For this review, use the dimensioned drawing (mm, ordinates from the lowest corner) and the shaded views. A direction names the side the tool comes from. Give positions to 0.01 mm unless a question says otherwise; leave off trailing zeros. Loops run counter-clockwise (first coordinate to the right, second up) from the corner with the lowest first, then second, coordinate; pieces in that order, holes last. Notation, with made-up numbers: M 64.25,-14.5 L 112.25,-14.5 A19 ccw 112.25,15.5 Z; hole C 39.25,-30.75 d1. An arc over 180 degrees is marked long. Return JSON: item names as keys, results as strings.
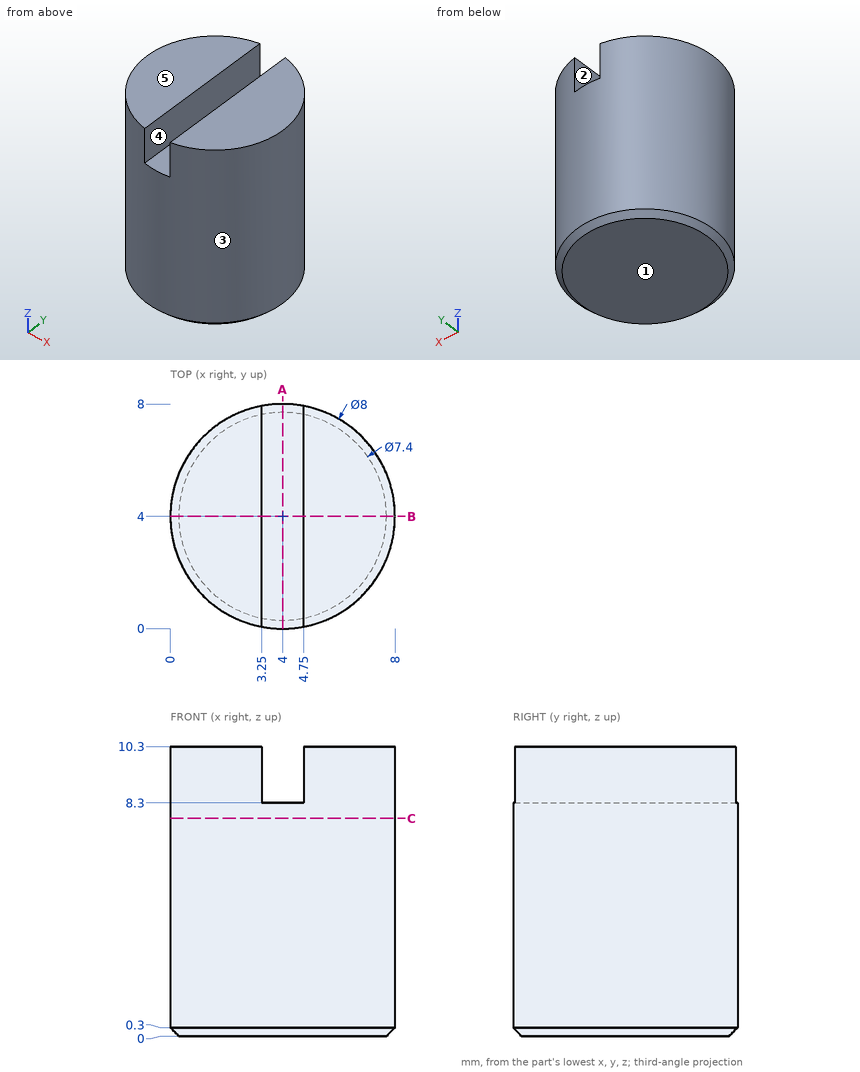
1) Wall thickness on L1, parallel to X at y = 2.5, z = 9; L2, parallel to Y at x = 3.25, z = 2.25; L3, parallel to Z at x = 3.5, y = 2.25: over which ranges is each line inside the solid? List them lowest first. Write a range as from..to.
From the geometry:
{"L1": "0.29..3.25, 4.75..7.71", "L2": "0.07..7.93", "L3": "0..8.3"}
2) Consider section C-C on z = 7.75. Write out the cut boundary in (x, y), then the cut area to 3 significant figures.
From the geometry:
{"outline": "C 4,4 d8", "area": "50.3 mm²"}
3) Insertion check: pin 1 (1 mm diameter, centred on x = 1.5, z = 1.5, fed in from -Y); pin 2 (0.6 mm diameter, centred on y = 2, z = 9, fed in from -X); pin 3 (0.6 mm diameter, centred on y = 3, z = 9.5, fed in from +X). Each pin has a flat end and moves straight along its axis. Give the tip position at first contact, or say it passes through.
From the geometry:
{"pin 1": "y = 0.54", "pin 2": "x = 0.38", "pin 3": "x = 7.94"}
4) The part is to be moulded in two halves that separate along X. For the marked faces 3, 4 and 5, say which applies: released by +X, released by -X, zero draft, split by the parting line, or undercut.
From the geometry:
{"face 3": "split by the parting line", "face 4": "undercut", "face 5": "zero draft"}
5) Consider section A-A on x = 4. Write out the cut boundary in (y, z).
From the geometry:
{"outline": "M 0,0.3 L 0.3,0 L 7.7,0 L 8,0.3 L 8,8.3 L 0,8.3 Z"}
6) Consider section B-B on y = 4. Write out the cut boundary in (x, z).
From the geometry:
{"outline": "M 0,0.3 L 0.3,0 L 7.7,0 L 8,0.3 L 8,10.3 L 4.75,10.3 L 4.75,8.3 L 3.25,8.3 L 3.25,10.3 L 0,10.3 Z"}
7) Tool access review of the marked faces 1 and 2: name each direction out of +Z, -Z, +X, -X, +Y, -Y from which nothing blocks a thin tool from reaching the whole face with its end or side.
From the geometry:
{"face 1": "-Z, +X, -X, +Y, -Y", "face 2": "+Z, +Y, -Y"}
